CAD build for the part. Positions are in the model's coordinates, mm. Round coordinates to 2 decimals unless told otherwise and drop trailing zeros. Order: outer loops, then holes, each group sorted by start corner. A loop starts at its lowest first (then second) coordinate and runs counter-clockwise, first axis right, second up. Notation, with made-up numbers: (61.25, 85.5) -> (102.25, 85.5) arc R13 cw to (102.25, 110.5) -> close; hole circle Ø3 at (18.5, 29). An arc over 180 degrees is marked (long way). Return JSON: item names as keys, results as strings. Group by question number.
Q1. Cut at D-D (x = 10). Write the cut outline in (y, z).
Q2. Cut at A-A (x = 4). Write the cut outline in (y, z), then the cut area to 3 significant figures.
Q3. Probe line 1 along X through (y, z) = (-3, 0.9); line 2 along X through (y, z) = (-2, 2.95); line 3 along Y through (x, z) = (3, 2.7). List the from-to ranges inside material, lowest first.
Q4. Cut at C-C (z = 1.9). Count the separate pieces of the cut face and the enclosed holes in it, then the cut area to 3 significant figures.
Q5. Mould opens along Y. For faces 1 (the cylindrical face through (0.86, -5.1, 2.03)), 2 (the flat face through (7, 0, 2)), 3 (the flat face through (7, -3, 0)), 4 (the cylindrical face through (9.89, -1.99, 1.97)) say: +Y half, -Y half, draft (parallel to the pull), parting line (faces both ways), or undercut.
Q6. Cut at B-B (y = -2.35). Write the cut outline in (x, z), then the cut area to 3 significant figures.
from build123d import *

# Parameters (mm, degrees)
SKETCH1_W               = 14
SKETCH1_H               = 6
BOSS_EXTRUDE1_DEPTH     = 4
CUT_EXTRUDE1_DEPTH      = 16.748015748
CUT_EXTRUDE1_DEPTH_BACK = 16.748015748
SKETCH2_R               = 1.3
SKETCH2_R_2             = 1.5
FILLET1_R               = 3


with BuildPart() as part:
    # Sketch1 → Boss-Extrude1 (new body)
    with BuildSketch(Plane.XY):
        with Locations((7, -3)):
            Rectangle(SKETCH1_W, SKETCH1_H)
    extrude(amount=BOSS_EXTRUDE1_DEPTH)

    # Sketch2 → Cut-Extrude1 (cut, two sides: drawn at the far end of the back side and taken through both)
    with BuildSketch(Plane.XY.offset(4).offset(-CUT_EXTRUDE1_DEPTH_BACK)):
        with Locations((3, -3)):
            Circle(SKETCH2_R)
        with Locations((11, -3)):
            Circle(SKETCH2_R_2)
    extrude(amount=CUT_EXTRUDE1_DEPTH + CUT_EXTRUDE1_DEPTH_BACK, mode=Mode.SUBTRACT)

    # Fillet1
    fillet1_edges = [part.edges().sort_by_distance(p)[0] for p in [
        (14, -6, 2),
        (14, 0, 2),
        (0, -6, 2),
        (0, 0, 2),
    ]]
    fillet(fillet1_edges, radius=FILLET1_R - 0.0001)  # a hair under: the kernel refuses the full size


solid = part.part
Solution:
{
 "1": {"outline": "(-6, 0) -> (-4.12, 0) -> (-4.12, 4) -> (-6, 4) -> close; (-1.88, 0) -> (0, 0) -> (0, 4) -> (-1.88, 4) -> close"},
 "2": {"outline": "(-6, 0) -> (-3.83, 0) -> (-3.83, 4) -> (-6, 4) -> close; (-2.17, 0) -> (0, 0) -> (0, 4) -> (-2.17, 4) -> close", "area": "17.4 mm²"},
 "3": {"line 1": "x = 0 to 1.7, 4.3 to 9.5, 12.5 to 14", "line 2": "x = 0.17 to 2.17, 3.83 to 9.88, 12.12 to 13.83", "line 3": "y = -6 to -4.3, -1.7 to 0"},
 "4": {"separate pieces": "1", "enclosed holes": "2", "area": "63.9 mm²"},
 "5": {"face 1": "-Y half", "face 2": "+Y half", "face 3": "draft", "face 4": "undercut"},
 "6": {"outline": "(0.07, 0) -> (1.87, 0) -> (1.87, 4) -> (0.07, 4) -> close; (4.13, 0) -> (9.65, 0) -> (9.65, 4) -> (4.13, 4) -> close; (12.35, 0) -> (13.93, 0) -> (13.93, 4) -> (12.35, 4) -> close", "area": "35.6 mm²"}
}
